For this review, take the finished solid that the model builds, in its own axes (mm). Face numbers are marked on the shaded views. A direction names the side the tool comes from. Coordinates: 2 decimals unless noted, no trailing zeros. Write each loop counter-clockwise with the first axis right and the second up, starting at its lowest first coordinate (ties: lowest second). Pieces come first, ordered by that corner, then holes.
```python
from build123d import *

# Parameters (mm, degrees)
SKETCH1_W                   = 127
SKETCH1_H                   = 127
BOSS_EXTRUDE1_DEPTH         = 12.7
SKETCH3_R                   = 15.875
BOSS_EXTRUDE2_DEPTH         = 3.175
F_1_4_0_25_DIAMETER_HOLE1_D = 6.35
F_1_4_0_25_DIAMETER_HOLE2_D = 6.35


with BuildPart() as part:
    # Sketch1 → Boss-Extrude1 (new body)
    with BuildSketch(Plane(origin=(0, 0, 0), x_dir=(1, 0, 0), z_dir=(0, 1, 0))):
        Rectangle(SKETCH1_W, SKETCH1_H)
    extrude(amount=BOSS_EXTRUDE1_DEPTH)

    # Sketch3 → Boss-Extrude2 (add)
    with BuildSketch(Plane(origin=(0, 12.7, 0), x_dir=(1, 0, 0), z_dir=(0, 1, 0))):
        with Locations(Location((0, 0, 0), (0, 0, 270))):
            Circle(SKETCH3_R)
    extrude(amount=BOSS_EXTRUDE2_DEPTH)

    # 1/4 (0.25) Diameter Hole1 (through all)
    with Locations(Plane(origin=(0, 12.7, 0), x_dir=(1, 0, 0), z_dir=(0, 1, 0))):
        with Locations((10.331110734, 23.204054624), (25.4, 0), (10.331110734, -23.204054624)):
            Hole(F_1_4_0_25_DIAMETER_HOLE1_D / 2)

    # 1/4 (0.25) Diameter Hole2 (through all)
    with Locations(Plane(origin=(0, 12.7, 0), x_dir=(1, 0, 0), z_dir=(0, 1, 0))):
        with Locations((-28.575, 0)):
            Hole(F_1_4_0_25_DIAMETER_HOLE2_D / 2)


solid = part.part
```
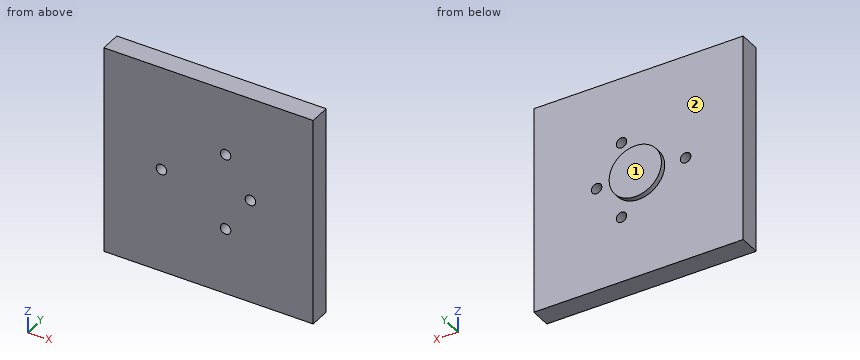
Q1. Add section C-C (x = 0). State the section outline as (y, z) points (3 decimals), then the cut area to 3 significant figures.
Ans:
outline: (0, -63.5) - (12.7, -63.5) - (12.7, -15.875) - (15.875, -15.875) - (15.875, 15.875) - (12.7, 15.875) - (12.7, 63.5) - (0, 63.5) - close
area: 1,710 mm2
Q2. Clearance check with flat-ended pins moving along their axes: pin 1 Ø10 at (x, z) = (-28.575, 0) entering from +Y; pin 2 Ø12 at (x, z) = (44, -46) entering from -Y. State where each tip first meets the part, or that it passes through.
Ans:
pin 1: stops at y = 12.7
pin 2: stops at y = 0
Q3. Add section D-D (z = 30). State the section outline as (x, y) points, then the cut area to 3 significant figures.
Ans:
outline: (-63.5, 0) - (63.5, 0) - (63.5, 12.7) - (-63.5, 12.7) - close
area: 1,610 mm2
Q4. Add section B-B (z = 0). State the section outline as (x, y) points (3 decimals).
Ans:
outline: (-63.5, 0) - (-31.75, 0) - (-31.75, 12.7) - (-63.5, 12.7) - close; (-25.4, 0) - (22.225, 0) - (22.225, 12.7) - (15.875, 12.7) - (15.875, 15.875) - (-15.875, 15.875) - (-15.875, 12.7) - (-25.4, 12.7) - close; (28.575, 0) - (63.5, 0) - (63.5, 12.7) - (28.575, 12.7) - close
Q5. Add section A-A (x = 25.4). State the section outline as (y, z) points (3 decimals), then the cut area to 3 significant figures.
Ans:
outline: (0, -63.5) - (12.7, -63.5) - (12.7, -3.175) - (0, -3.175) - close; (0, 3.175) - (12.7, 3.175) - (12.7, 63.5) - (0, 63.5) - close
area: 1,530 mm2
Q6. Tool access review of the marked faces 1 and 2: name each direction out of +Z, -Z, +X, -X, +Y, -Y from which nothing blocks a thin tool from reaching the whole face with its end or side.
Ans:
face 1: +Z, -Z, +X, -X, +Y
face 2: +Y
Q7. For probe 1 along Z at (x, y) = (25.4, 6) (3 decimals); probe 2 along Y at (x, z) = (15, 26.5); probe 3 along X at (y, z) = (12.75, 0.5), list the stretches that pass through material, from the lowest coordinate up.
Ans:
probe 1: z = -63.5 to -3.175, 3.175 to 63.5
probe 2: y = 0 to 12.7
probe 3: x = -15.87 to 15.87
